from build123d import *

# Parameters (mm, degrees)
SKETCH1_W           = 114.808
SKETCH1_H           = 23.114
BOSS_EXTRUDE1_DEPTH = 5.334
FILLET1_R           = 6.35
SKETCH3_W           = 43.18
SKETCH3_H           = 9.401705223
SKETCH3_W_2         = 44.45
CUT_EXTRUDE2_DEPTH  = 474.106416887


with BuildPart() as part:
    # Sketch1 → Boss-Extrude1 (new body)
    with BuildSketch(Plane(origin=(0, 0, 0), x_dir=(1, 0, 0), z_dir=(0, 1, 0))):
        with Locations((-373.645654051, 183.372284322)):
            Rectangle(SKETCH1_W, SKETCH1_H)
    extrude(amount=BOSS_EXTRUDE1_DEPTH)

    # Fillet1
    fillet1_edges = [part.edges().sort_by_distance(p)[0] for p in [
        (-431.049654051, 2.667, -194.929284322),
    ]]
    fillet(fillet1_edges, radius=FILLET1_R)

    # Sketch3 → Cut-Extrude2 (cut, through all)
    with BuildSketch(Plane(origin=(0, 5.334, 0), x_dir=(1, 0, 0), z_dir=(0, 1, 0))):
        with Locations((-409.459654051, 176.516136934)):
            Rectangle(SKETCH3_W, SKETCH3_H)
        with Locations((-338.466654051, 176.516136934)):
            Rectangle(SKETCH3_W_2, SKETCH3_H)
    extrude(amount=-CUT_EXTRUDE2_DEPTH, mode=Mode.SUBTRACT)


solid = part.part
Can you work these out from the model? Positions are in its coordinate system, mm. A direction names the side the tool comes from. Coordinates: 2 decimals unless noted, no trailing zeros. Loops run counter-clockwise (first coordinate to the right, second up) from the corner with the lowest first, then second, coordinate; pieces in that order, holes last. Notation, with made-up numbers: (-2, 4.5) - (47, 4.5) arc R32 cw to (47, 32.5) - close; hole circle Ø6 at (63.25, 45.5). An arc over 180 degrees is marked (long way). Answer as a JSON object with one key per item and string values. Group by question number.
Item 1: If we section it at B-B (z = -178.5): List the corners of the cut face in (x, y) for me.
Item 2: If I drill on L1, parallel to X at y = 5, z = -177; L2, parallel to Z at x = -424, y = 4.25; L3, parallel to X at y = 0.8, z = -190.5, over which ranges is the centre line in solid material (lowest first)? Write a range as from..to.
Item 3: For pin 1 (2 mm diameter, centred on x = -355, z = -186.5, fed in from -Y); pin 2 (2.5 mm diameter, centred on y = 2, z = -176.5, fed in from -X); pin 3 (12 mm diameter, centred on x = -341.5, z = -174.5, fed in from +Y); pin 4 (2.5 mm diameter, centred on x = -405, y = 2, fed in from +Z), each with a flat end and sliding along its axis, tell me the tip position at first contact or that it passes through.
Item 4: If we section it at A-A (y = 4): List the corners of the cut face in (x, z) for me.
Item 5: If we section it at C-C (x = -422.5): List the corners of the cut face in (y, z) for me, plus the area to 3 significant figures.
Item 6: On a 3-axis mill with a long thin cutter (end or side, diameter ignored), from which of +Z, -Z, +X, -X, +Y, -Y can I reach the whole of each face in a straight line? I mean faces 1 (the face through (-339, 3, -181.217)), 2 (the face through (-316.242, 3, -188)), 3 (the face through (-387.87, 3, -176)). Say none if no direction works.
Returned:
{
 "1": {"outline": "(-387.87, 0) - (-360.69, 0) - (-360.69, 5.33) - (-387.87, 5.33) - close"},
 "2": {"L1": "x = -387.87..-360.69", "L2": "z = -194.93..-181.22", "L3": "x = -430.75..-316.24"},
 "3": {"pin 1": "stops at y = 0", "pin 2": "stops at x = -387.87", "pin 3": "passes through", "pin 4": "stops at z = -181.22"},
 "4": {"outline": "(-431.05, -188.58) arc R6.35 ccw to (-424.7, -194.93) - (-316.24, -194.93) - (-316.24, -181.22) - (-360.69, -181.22) - (-360.69, -171.82) - (-387.87, -171.82) - (-387.87, -181.22) - (-431.05, -181.22) - close"},
 "5": {"outline": "(0, -194.93) - (5.33, -194.93) - (5.33, -181.22) - (0, -181.22) - close", "area": "73.1 mm²"},
 "6": {"face 1": "+Z, +X, +Y, -Y", "face 2": "+Z, -Z, +X, +Y, -Y", "face 3": "+Z, -X, +Y, -Y"}
}
